Could you check a few things on this model? Use its own coordinates, in mm. Round coordinates to 2 decimals unless told otherwise and drop trailing zeros. Loops run counter-clockwise (first coordinate to the right, second up) from the corner with the lowest first, then second, coordinate; pieces in that order, holes last.
from build123d import *

# Parameters (mm, degrees)
SKETCH3_W               = 25.4
SKETCH3_H               = 12.7
SKETCH3_W_2             = 22.225
SKETCH3_H_2             = 9.525
BOSS_EXTRUDE1_DEPTH     = 152.4
SKETCH4_R               = 2
CUT_EXTRUDE1_DEPTH      = 1.5875
SKETCH5_R               = 1.500419334
CUT_EXTRUDE2_DEPTH      = 1.5875
CUT_EXTRUDE3_DEPTH      = 154.454683865
CUT_EXTRUDE3_DEPTH_BACK = 2.54
M4X0_7_TAPPED_HOLE1_D   = 3.3


with BuildPart() as part:
    # Sketch3 → Boss-Extrude1 (new body)
    with BuildSketch(Plane.XY):
        Rectangle(SKETCH3_W, SKETCH3_H)
        Rectangle(SKETCH3_W_2, SKETCH3_H_2, mode=Mode.SUBTRACT)
    extrude(amount=BOSS_EXTRUDE1_DEPTH)

    # Sketch4 → Cut-Extrude1 (cut)
    with BuildSketch(Plane(origin=(0, 6.35, 0), x_dir=(1, 0, 0), z_dir=(0, 1, 0))):
        with Locations(Location((0, -141.4, 0), (0, 0, 270))):
            Circle(SKETCH4_R)
    extrude(amount=-CUT_EXTRUDE1_DEPTH, mode=Mode.SUBTRACT)

    # Sketch5 → Cut-Extrude2 (cut)
    with BuildSketch(Plane.XZ.offset(6.35)):
        with Locations((-8, 141.4)):
            Circle(SKETCH5_R)
        with Locations((0, 149.4)):
            Circle(SKETCH5_R)
        with Locations((8, 141.4)):
            Circle(SKETCH5_R)
    extrude(amount=-CUT_EXTRUDE2_DEPTH, mode=Mode.SUBTRACT)

    # Sketch6 → Cut-Extrude3 (cut, two sides: drawn at the far end of the back side and taken through both)
    with BuildSketch(Plane.XZ.offset(6.35).offset(-CUT_EXTRUDE3_DEPTH_BACK)):
        Polygon((-5, 469.248822712), (-5, 152.4), (-5, 136.4), (5, 136.4), (5, 152.4), (5, 469.248822712), (5, 1102.946468137), (-5, 1102.946468137), align=None)
    extrude(amount=CUT_EXTRUDE3_DEPTH + CUT_EXTRUDE3_DEPTH_BACK, mode=Mode.SUBTRACT)

    # M4x0.7 Tapped Hole1 (through all)
    with Locations(Plane(origin=(0, -6.35, 0), x_dir=(-1, 0, 0), z_dir=(0, -1, 0))):
        with Locations((0, -20.199999986), (0, -7.5)):
            Hole(M4X0_7_TAPPED_HOLE1_D / 2)


solid = part.part
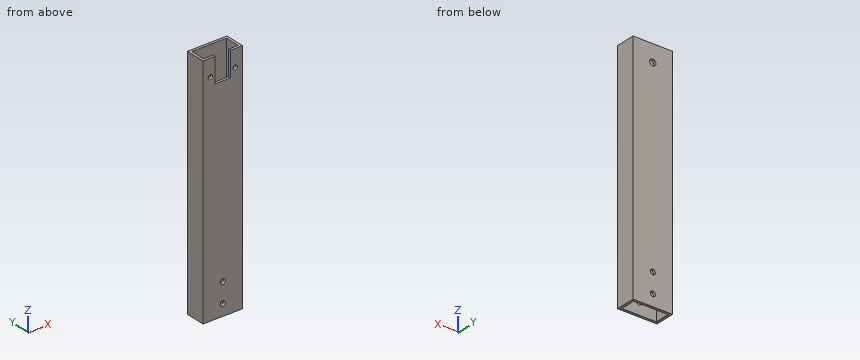
Item 1: If we section it at D-D, the plane z = 40: Please give me the cut outline in (x, y).
Results list:
outline: (-12.7, -6.35) - (12.7, -6.35) - (12.7, 6.35) - (-12.7, 6.35) - close; hole (-11.11, -4.76) - (11.11, -4.76) - (11.11, 4.76) - (-11.11, 4.76) - close
Item 2: If we section it at C-C, the plane y = -2.25: Please give me the cut outline in (x, z).
Results list:
outline: (-12.7, 0) - (-11.11, 0) - (-11.11, 152.4) - (-12.7, 152.4) - close; (11.11, 0) - (12.7, 0) - (12.7, 152.4) - (11.11, 152.4) - close
Item 3: If we section it at A-A, the plane z = 7.5: Please give me the cut outline in (x, y), then the cut area to 3 significant figures.
Results list:
outline: (-12.7, -6.35) - (-1.65, -6.35) - (-1.65, -4.76) - (-11.11, -4.76) - (-11.11, 4.76) - (-1.65, 4.76) - (-1.65, 6.35) - (-12.7, 6.35) - close; (1.65, -6.35) - (12.7, -6.35) - (12.7, 6.35) - (1.65, 6.35) - (1.65, 4.76) - (11.11, 4.76) - (11.11, -4.76) - (1.65, -4.76) - close
area: 100 mm2
Item 4: If we section it at B-B, the plane x = 8: Please give me the cut outline in (y, z).
Results list:
outline: (-6.35, 0) - (-4.76, 0) - (-4.76, 139.9) - (-6.35, 139.9) - close; (-6.35, 142.9) - (-4.76, 142.9) - (-4.76, 152.4) - (-6.35, 152.4) - close; (4.76, 0) - (6.35, 0) - (6.35, 152.4) - (4.76, 152.4) - close
Item 5: Will these pins go through, and if not, where does the flat tip stop? pin 1 (4 mm diameter, centred on x = 0, z = 20.2, fed in from +Y); pin 2 (2.5 mm diameter, centred on x = 8, z = 141.4, fed in from -Y); pin 3 (1.7 mm diameter, centred on x = -1.5, y = -5.5, fed in from +Z).
Results list:
pin 1: stops at y = 6.35
pin 2: stops at y = 4.76
pin 3: stops at z = 136.4
Item 6: If I drill on line 1 along Z through (x, y) = (0, -5.4); line 2 along X through (y, z) = (-5.45, 141.4); line 3 along Y through (x, z) = (-8.5, 137.5), over which ranges is the centre line in solid material (lowest first)?
Results list:
line 1: z = 0 to 5.85, 9.15 to 18.55, 21.85 to 136.4
line 2: x = -12.7 to -9.5, -6.5 to -5, 5 to 6.5, 9.5 to 12.7
line 3: y = -6.35 to -4.76, 4.76 to 6.35
